from build123d import *

# Parameters (mm, degrees)
SKETCH1_W           = 20.5
SKETCH1_H           = 30.5
BOSS_EXTRUDE1_DEPTH = 1.5
SKETCH2_W           = 15
SKETCH2_H           = 11.5
BOSS_EXTRUDE2_DEPTH = 3
SKETCH3_W           = 3
SKETCH3_H           = 10
BOSS_EXTRUDE3_DEPTH = 10
SKETCH4_W           = 20.5
SKETCH4_H           = 7.5
BOSS_EXTRUDE4_DEPTH = 10
SKETCH5_W           = 4.125
SKETCH5_H           = 5
CUT_EXTRUDE1_DEPTH  = 3
CHAMFER1_SIZE       = 2.5
CHAMFER1_SIZE2      = 2
CHAMFER2_SIZE       = 3.5
CHAMFER2_SIZE2      = 1
SKETCH6_R           = 1.5
CUT_EXTRUDE2_DEPTH  = 3
SKETCH8_W           = 17.5
SKETCH8_H           = 28.7
BOSS_EXTRUDE5_DEPTH = 2.5


with BuildPart() as part:
    # Sketch1 → Boss-Extrude1 (new body)
    with BuildSketch(Plane(origin=(0, 0, 0), x_dir=(1, 0, 0), z_dir=(0, 1, 0))):
        Rectangle(SKETCH1_W, SKETCH1_H)
    extrude(amount=BOSS_EXTRUDE1_DEPTH)

    # Sketch2 → Boss-Extrude2 (add)
    with BuildSketch(Plane(origin=(0, 1.5, 0), x_dir=(1, 0, 0), z_dir=(0, 1, 0))):
        with Locations((0, -16.5)):
            Rectangle(SKETCH2_W, SKETCH2_H)
    extrude(amount=BOSS_EXTRUDE2_DEPTH)

    # Sketch3 → Boss-Extrude3 (add)
    with BuildSketch(Plane(origin=(0, 1.5, 0), x_dir=(1, 0, 0), z_dir=(0, 1, 0))):
        with Locations((6.25, -0.25)):
            Rectangle(SKETCH3_W, SKETCH3_H)
    extrude(amount=BOSS_EXTRUDE3_DEPTH)

    # Sketch4 → Boss-Extrude4 (add)
    with BuildSketch(Plane(origin=(0, 1.5, 0), x_dir=(1, 0, 0), z_dir=(0, 1, 0))):
        with Locations((0, 11.5)):
            Rectangle(SKETCH4_W, SKETCH4_H)
    extrude(amount=BOSS_EXTRUDE4_DEPTH)

    # Sketch5 → Cut-Extrude1 (cut)
    with BuildSketch(Plane(origin=(0, 0, -15.25), x_dir=(-1, 0, 0), z_dir=(0, 0, -1))):
        with Locations((-7.6875, 5)):
            Rectangle(SKETCH5_W, SKETCH5_H)
        with Locations((-2.5625, 5)):
            Rectangle(SKETCH5_W, SKETCH5_H)
        with Locations((2.5625, 5)):
            Rectangle(SKETCH5_W, SKETCH5_H)
        with Locations((7.6875, 5)):
            Rectangle(SKETCH5_W, SKETCH5_H)
    extrude(amount=-CUT_EXTRUDE1_DEPTH, mode=Mode.SUBTRACT)

    # Chamfer1
    chamfer1_edges = [part.edges().sort_by_distance(p)[0] for p in [
        (0, 11.5, -7.75),
    ]]
    chamfer1_side = [part.faces().sort_by_distance(p)[0] for p in [
        (0, 6.5, -7.75),
    ]]
    chamfer(chamfer1_edges, length=CHAMFER1_SIZE, length2=CHAMFER1_SIZE2, reference=chamfer1_side[0])

    # Chamfer2
    chamfer2_edges = [part.edges().sort_by_distance(p)[0] for p in [
        (0, 11.5, -15.25),
    ]]
    chamfer2_side = [part.faces().sort_by_distance(p)[0] for p in [
        (0, 6.153752039, -15.25),
    ]]
    chamfer(chamfer2_edges, length=CHAMFER2_SIZE, length2=CHAMFER2_SIZE2, reference=chamfer2_side[0])

    # Sketch6 → Cut-Extrude2 (cut)
    with BuildSketch(Plane(origin=(0, 11.5, 0), x_dir=(1, 0, 0), z_dir=(0, 1, 0))):
        with Locations((-7.5, 11.75)):
            Circle(SKETCH6_R)
        with Locations((-2.5, 11.75)):
            Circle(SKETCH6_R)
        with Locations((2.5, 11.75)):
            Circle(SKETCH6_R)
        with Locations((7.5, 11.75)):
            Circle(SKETCH6_R)
    extrude(amount=-CUT_EXTRUDE2_DEPTH, mode=Mode.SUBTRACT)

    # Sketch8 → Boss-Extrude5 (add)
    with BuildSketch(Plane.XZ):
        Rectangle(SKETCH8_W, SKETCH8_H)
    extrude(amount=BOSS_EXTRUDE5_DEPTH)


solid = part.part
Build history of the part. All positions in model axes, mm. A direction names the side the tool comes from. Round coordinates to 2 decimals unless told otherwise and drop trailing zeros. Write each loop counter-clockwise with the first axis right and the second up, starting at its lowest first coordinate (ties: lowest second). Pieces come first, ordered by that corner, then holes. Notation, with made-up numbers: (87.25, -1) -> (131.25, -1) arc R26 ccw to (131.25, 22) -> close; hole circle Ø3 at (65, 2.25). An arc over 180 degrees is marked (long way). Use one line per item in the form item = value.
Q1. Tool access for faces 1 (the flat face through (0, 5, -7.75)), 2 (the flat face through (-8.75, -1, 0)), 3 (the cylindrical face through (-1.114, 10.021, -11.175)), 4 (the flat face through (6, 11.5, 0)), 5 (the flat face through (0.5, 5, -14)): list every direction of +Z, -Z, +X, -X, +Y, -Y with a clear straight run to the whole face (end or side of a thin tool).
Conclusion:
face_1 = +X, -X, +Y
face_2 = +Z, -Z, -X, -Y
face_3 = +Y
face_4 = +Z, -Z, +X, -X, +Y
face_5 = -Z
Q2. Drop flat-ended pins along their axis: P1, Ø1, axis at y = 2.5, z = 4.5, coming from the -X side; P2, Ø2.5, axis at x = -7.5, z = -11.75, coming from the +Y side; P3, Ø1.5, axis at y = 3, z = 16.5, coming from the +X side. Give the stop position or say it passes through.
Conclusion:
P1 = 4.75
P2 = 8.5
P3 = 7.5
Q3. Two-plate mould, pull along X, no slides. Class faces 6 (the flat face through (7.5, 3, 17)), 7 (the flat face through (3, 2.5, -14)), 8 (the flat face through (4.75, 6, 0)): released by +X, released by -X, zero draft, split by the parting line, or undercut.
Conclusion:
face_6 = released by +X
face_7 = undercut
face_8 = released by -X
Q4. Band-saw the part on C-C, the plane x = 2.5. Write the cut outline in (y, z).
Conclusion:
outline = (-2.5, -14.35) -> (0, -14.35) -> (0, -15.25) -> (2.5, -15.25) -> (2.5, -12.25) -> (7.5, -12.25) -> (7.5, -15.25) -> (8, -15.25) -> (11.5, -14.25) -> (11.5, -13.25) -> (8.5, -13.25) -> (8.5, -10.25) -> (11.5, -10.25) -> (11.5, -9.75) -> (9, -7.75) -> (1.5, -7.75) -> (1.5, 10.75) -> (4.5, 10.75) -> (4.5, 22.25) -> (1.5, 22.25) -> (1.5, 15.25) -> (0, 15.25) -> (0, 14.35) -> (-2.5, 14.35) -> close
Q5. Band-saw the part on B-B, the plane y = 3. Write the cut outline in (x, z) (3 decimals).
Conclusion:
outline = (-10.25, -15.25) -> (-9.75, -15.25) -> (-9.75, -12.25) -> (-5.625, -12.25) -> (-5.625, -15.25) -> (-4.625, -15.25) -> (-4.625, -12.25) -> (-0.5, -12.25) -> (-0.5, -15.25) -> (0.5, -15.25) -> (0.5, -12.25) -> (4.625, -12.25) -> (4.625, -15.25) -> (5.625, -15.25) -> (5.625, -12.25) -> (9.75, -12.25) -> (9.75, -15.25) -> (10.25, -15.25) -> (10.25, -7.75) -> (-10.25, -7.75) -> close; (-7.5, 10.75) -> (7.5, 10.75) -> (7.5, 22.25) -> (-7.5, 22.25) -> close; (4.75, -4.75) -> (7.75, -4.75) -> (7.75, 5.25) -> (4.75, 5.25) -> close
Q6. Drill centre lines: L1, parallel to X at y = 10.85, z = -11.75; L2, parallel to Z at x = 3, y = 3.5; L3, parallel to Z at x = 7.5, y = 9.7. Where is each one in solid material? Low to high.
Conclusion:
L1 = -10.25 to -9, -6 to -4, -1 to 1, 4 to 6, 9 to 10.25
L2 = -12.25 to -7.75, 10.75 to 22.25
L3 = -14.76 to -13.25, -10.25 to -8.31, -4.75 to 5.25
Q7. Band-saw the part on A-A, the plane y = 9.75. Write the cut outline in (x, z), then the cut area to 3 significant figures.
Conclusion:
outline = (-10.25, -14.75) -> (10.25, -14.75) -> (10.25, -8.35) -> (-10.25, -8.35) -> close; (4.75, -4.75) -> (7.75, -4.75) -> (7.75, 5.25) -> (4.75, 5.25) -> close; hole circle Ø3 at (-7.5, -11.75); hole circle Ø3 at (-2.5, -11.75); hole circle Ø3 at (2.5, -11.75); hole circle Ø3 at (7.5, -11.75)
area = 133 mm²
Q8. Band-saw the part on D-D, the plane z = -11.75. Write the cut outline in (x, y).
Conclusion:
outline = (-10.25, 0) -> (-8.75, 0) -> (-8.75, -2.5) -> (8.75, -2.5) -> (8.75, 0) -> (10.25, 0) -> (10.25, 11.5) -> (9, 11.5) -> (9, 8.5) -> (6, 8.5) -> (6, 11.5) -> (4, 11.5) -> (4, 8.5) -> (1, 8.5) -> (1, 11.5) -> (-1, 11.5) -> (-1, 8.5) -> (-4, 8.5) -> (-4, 11.5) -> (-6, 11.5) -> (-6, 8.5) -> (-9, 8.5) -> (-9, 11.5) -> (-10.25, 11.5) -> close
